Could you check a few things on this model? Use its own coordinates, in mm. Face numbers are marked on the shaded views. A direction names the side the tool comes from. Give positions to 0.01 mm unless a question says otherwise; leave off trailing zeros. Write each loop counter-clockwise with the first axis right and the second up, starting at its lowest first coordinate (ties: lowest second). Pieces come first, ordered by that corner, then holes. Notation, with made-up numbers: (87, 79.5) - (120, 79.5) arc R18 ccw to (120, 86.5) - close; hole circle Ø7 at (46, 25). An arc over 180 degrees is marked (long way). Answer in a Markdown table with one row per item.
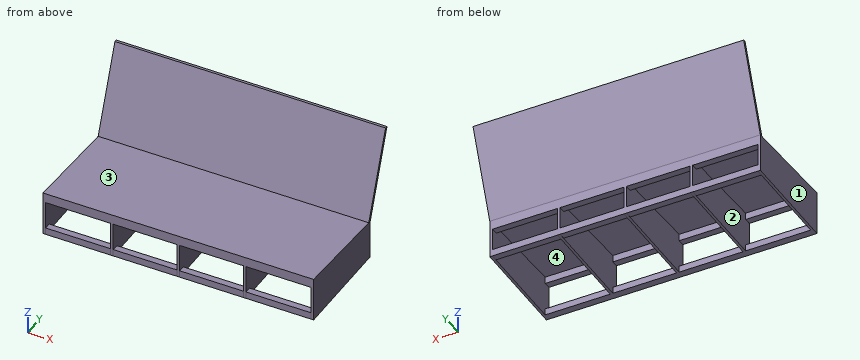
from build123d import *

# Parameters (mm, degrees)
F0_W       = 2000
F0_H       = 750
F1_DEPTH   = 19
F2_W       = 19
F2_H       = 750
F3_DEPTH   = 300
F4_SIZE2   = 39.99999
F4_SIZE    = 749.99999
F4_2_SIZE2 = 39.99999
F4_2_SIZE  = 749.99999
F4_3_SIZE2 = 39.99999
F4_3_SIZE  = 749.99999
F4_4_SIZE2 = 39.99999
F4_4_SIZE  = 749.99999
F4_5_SIZE2 = 39.99999
F4_5_SIZE  = 749.99999
F6_DEPTH   = 2000
F10_W      = 481
F10_H      = 50
F9_W       = 471.5
F9_H       = 50
F8_W       = 471.5
F8_H       = 50
F7_W       = 481
F7_H       = 50
F11_DEPTH  = 50
F12_W      = 50
F12_H      = 50
F13_DEPTH  = 2000


# Not quite as in the source:
# - a fillet or chamfer is up to 0.001 mm smaller than in the source, because OpenCascade refuses the exact size
# - ends of sketch curves that miss each other by under 0.0002 mm in the source are joined


with BuildPart() as f1:
    # F0 (on Top) → F1 (new body)
    with BuildSketch(Plane.XY):
        Rectangle(F0_W, F0_H)
    extrude(amount=F1_DEPTH)

    # F2 (on face) → F3 (join)
    with BuildSketch(Plane(origin=(0, 0, 0), x_dir=(1, 0, 0), z_dir=(0, 0, -1))):
        with Locations((-990.5, 0)):
            Rectangle(F2_W, F2_H)
        with Locations((-490.5, 0)):
            Rectangle(F2_W, F2_H)
        Rectangle(F2_W, F2_H)
        with Locations((490.5, 0)):
            Rectangle(F2_W, F2_H)
        with Locations((990.5, 0)):
            Rectangle(F2_W, F2_H)
    extrude(amount=F3_DEPTH)

    # F4 (size 750 and 40 in the source; OpenCascade refuses exactly that, so slightly less here)
    f4_edges = [f1.edges().sort_by_distance(p)[0] for p in [
        (990.5, 375, -300),
    ]]
    f4_side = f1.faces().sort_by_distance((990.5, 0, -300))[0]
    chamfer(f4_edges, length=F4_SIZE, length2=F4_SIZE2, reference=f4_side)

    # F4#2 (size 750 and 40 in the source; OpenCascade refuses exactly that, so slightly less here)
    f4_2_edges = [f1.edges().sort_by_distance(p)[0] for p in [
        (490.5, 375, -300),
    ]]
    f4_2_side = f1.faces().sort_by_distance((490.5, 0, -300))[0]
    chamfer(f4_2_edges, length=F4_2_SIZE, length2=F4_2_SIZE2, reference=f4_2_side)

    # F4#3 (size 750 and 40 in the source; OpenCascade refuses exactly that, so slightly less here)
    f4_3_edges = [f1.edges().sort_by_distance(p)[0] for p in [
        (0, 375, -300),
    ]]
    f4_3_side = f1.faces().sort_by_distance((0, 0, -300))[0]
    chamfer(f4_3_edges, length=F4_3_SIZE, length2=F4_3_SIZE2, reference=f4_3_side)

    # F4#4 (size 750 and 40 in the source; OpenCascade refuses exactly that, so slightly less here)
    f4_4_edges = [f1.edges().sort_by_distance(p)[0] for p in [
        (-490.5, 375, -300),
    ]]
    f4_4_side = f1.faces().sort_by_distance((-490.5, 0, -300))[0]
    chamfer(f4_4_edges, length=F4_4_SIZE, length2=F4_4_SIZE2, reference=f4_4_side)

    # F4#5 (size 750 and 40 in the source; OpenCascade refuses exactly that, so slightly less here)
    f4_5_edges = [f1.edges().sort_by_distance(p)[0] for p in [
        (-990.5, 375, -300),
    ]]
    f4_5_side = f1.faces().sort_by_distance((-990.5, 0, -300))[0]
    chamfer(f4_5_edges, length=F4_5_SIZE, length2=F4_5_SIZE2, reference=f4_5_side)

    # F5 (on face) → F6 (join)
    with BuildSketch(Plane(origin=(-1000, 0, 0), x_dir=(0, -1, 0), z_dir=(-1, 0, 0))):
        Polygon((-597.3130931617, 629.8002035108), (-375, 19), (-356, 19), (-578.3130931617, 629.8002035108), align=None)
    extrude(amount=-F6_DEPTH)

    # F10 (on face) + F9 (on face) + F8 (on face) + F7 (on face) → F11 (join)
    with BuildSketch(Plane(origin=(0, 0, 0), x_dir=(1, 0, 0), z_dir=(0, 0, -1))):
        with Locations((-740.5, 350)):
            Rectangle(F10_W, F10_H)
        with Locations((-740.5, -350)):
            Rectangle(F10_W, F10_H)
    with BuildSketch(Plane(origin=(0, 0, 0), x_dir=(1, 0, 0), z_dir=(0, 0, -1))):
        with Locations((-245.25, -350)):
            Rectangle(F9_W, F9_H)
        with Locations((-245.25, 350)):
            Rectangle(F9_W, F9_H)
    with BuildSketch(Plane(origin=(0, 0, 0), x_dir=(1, 0, 0), z_dir=(0, 0, -1))):
        with Locations((245.25, 350)):
            Rectangle(F8_W, F8_H)
        with Locations((245.25, -350)):
            Rectangle(F8_W, F8_H)
    with BuildSketch(Plane(origin=(0, 0, 0), x_dir=(1, 0, 0), z_dir=(0, 0, -1))):
        with Locations((740.5, 350)):
            Rectangle(F7_W, F7_H)
        with Locations((740.5, -350)):
            Rectangle(F7_W, F7_H)
    extrude(amount=F11_DEPTH)

    # F12 (on face) → F13 (join)
    with BuildSketch(Plane(origin=(-1000, 0, 0), x_dir=(0, -1, 0), z_dir=(-1, 0, 0))):
        with Locations((-350, -235)):
            Rectangle(F12_W, F12_H)
        Polygon((325, -250), (325, -297.3333344978), (374.99999, -300), (375, -250), align=None)
    extrude(amount=-F13_DEPTH)


solid = f1.part
1) On a 3-axis mill with a long thin cutter (end or side, diameter ignored), from which of +Z, -Z, +X, -X, +Y, -Y can I reach the whole of each face in a straight line? I mean the marked faces 1, 2, 3 and 4. Say none if no direction works.
Check values:
| item | result |
|---|---|
| face 1 | +Z, -Z, -X, +Y, -Y |
| face 2 | none |
| face 3 | +Z, +X, -X, -Y |
| face 4 | -Z |
2) Imagine slicing it at B-B (z = -134.5). List the corners of the cut face in (x, y) for me, then the cut area to 4 significant figures.
Check values:
| item | result |
|---|---|
| outline | (-1000, -375) - (-981, -375) - (-981, 375) - (-1000, 375) - close; (-500, -375) - (-481, -375) - (-481, 375) - (-500, 375) - close; (-9.5, -375) - (9.5, -375) - (9.5, 375) - (-9.5, 375) - close; (481, -375) - (500, -375) - (500, 375) - (481, 375) - close; (981, -375) - (1000, -375) - (1000, 375) - (981, 375) - close |
| area | 71,250 mm2 |
3) Imagine slicing it at A-A (x = -322.5). List the corners of the cut face in (y, z) for me.
Check values:
| item | result |
|---|---|
| outline | (-375, -300) - (-325, -297.33) - (-325, -250) - (-375, -250) - close; (-375, -50) - (-325, -50) - (-325, 0) - (325, 0) - (325, -50) - (375, -50) - (375, 19) - (597.31, 629.8) - (578.31, 629.8) - (356, 19) - (-375, 19) - close; (325, -260) - (375, -260) - (375, -210) - (325, -210) - close |
4) Imagine slicing it at C-C (y = 278.5). List the corners of the cut face in (x, z) for me, then the cut area to 3 significant figures.
Check values:
| item | result |
|---|---|
| outline | (-1000, -265.15) - (-981, -265.15) - (-981, 0) - (-500, 0) - (-500, -265.15) - (-481, -265.15) - (-481, 0) - (-9.5, 0) - (-9.5, -265.15) - (9.5, -265.15) - (9.5, 0) - (481, 0) - (481, -265.15) - (500, -265.15) - (500, 0) - (981, 0) - (981, -265.15) - (1000, -265.15) - (1000, 19) - (-1000, 19) - close |
| area | 63,200 mm2 |
5) Imagine slicing it at D-D (z = 386). List the corners of the cut face in (x, y) for me.
Check values:
| item | result |
|---|---|
| outline | (-1000, 489.58) - (1000, 489.58) - (1000, 508.58) - (-1000, 508.58) - close |
6) If I drill on line 1 (X direction, y = -48, z = -131.5); line 2 (Y direction, x = -905, z = -42.5); line 3 (Z direction, x = 213.5, y = -259), over which ranges is the centre line in solid material (lowest first)?
Check values:
| item | result |
|---|---|
| line 1 | x = -1000 to -981, -500 to -481, -9.5 to 9.5, 481 to 500, 981 to 1000 |
| line 2 | y = -375 to -325, 325 to 375 |
| line 3 | z = 0 to 19 |
7) Will these pins go through, and if not, where does the flat tip stop? P1, Ø12, axis at x = -794.5, y = 3, coming from the -Z side; P2, Ø5, axis at x = 544, z = 145.5, coming from the +Y side; P3, Ø15, axis at x = -791, y = 360, coming from the -Z side; P4, Ø25, axis at x = 272, z = -245.5, coming from the -Y side.
Check values:
| item | result |
|---|---|
| P1 | stops at z = 0 |
| P2 | stops at y = 421.95 |
| P3 | stops at z = -260 |
| P4 | stops at y = -375 |
